Read the model definition and answer for the solid it produces. Units are mm, in the model's axes. A direction names the side the tool comes from. Coordinates: 2 decimals unless noted, no trailing zeros. Write each loop counter-clockwise with the first axis right and the second up, starting at its lowest first coordinate (ties: lowest second). Pieces come first, ordered by that corner, then holes. Notation, with made-up numbers: (41, 26) - (73, 26) arc R30 ccw to (73, 55) - close; hole circle Ø2 at (39, -21). An arc over 180 degrees is marked (long way). Use a Markdown table: item, result.
from build123d import *

# Parameters (mm, degrees)
ESBO_O1_W                  = 170
ESBO_O1_H                  = 30
RESSALTO_EXTRUS_O1_DEPTH   = 150
CORTE_EXTRUS_O1_DEPTH      = 222
CORTE_EXTRUS_O1_DEPTH_BACK = 36
RESSALTO_EXTRUS_O2_DEPTH   = 5
RESSALTO_EXTRUS_O3_DEPTH   = 5
ESBO_O4_W                  = 159.333333333
ESBO_O4_H                  = 140.588235294
CORTE_EXTRUS_O2_DEPTH      = 25
CORTE_EXTRUS_O3_DEPTH      = 31
CORTE_EXTRUS_O4_DEPTH      = 42
FILETE1_R                  = 10
CORTE_EXTRUS_O5_DEPTH      = 32
CORTE_EXTRUS_O6_START      = -15.72292277
CORTE_EXTRUS_O6_OUTLINE_R  = 3.95
CORTE_EXTRUS_O6_DEPTH      = 4.876648775
CORTE_EXTRUS_O7_START      = -132.751356438
CORTE_EXTRUS_O7_OUTLINE_R  = 3.95
CORTE_EXTRUS_O7_DEPTH      = 3.479370229
RESSALTO_EXTRUS_O6_DEPTH   = 17
RESSALTO_EXTRUS_O7_DEPTH   = 4
CORTE_EXTRUS_O8_DEPTH      = 21
F_3DSKETCH12_R             = 1.5
CORTE_EXTRUS_O9_DEPTH      = 14
CORTE_EXTRUS_O10_DEPTH     = 19
ESBO_O11_W                 = 17.407525744
ESBO_O11_H                 = 16.792397695
CORTE_EXTRUS_O11_DEPTH     = 10
CORTE_EXTRUS_O12_DEPTH     = 20
CORTE_EXTRUS_O13_DEPTH     = 14


# Read off the part's stored shape, not the designer's step: Corte-extrusão6, Corte-extrusão7
with BuildPart() as part:
    # Esboço1 → Ressalto-extrusão1 (new body)
    with BuildSketch(Plane(origin=(0, 0, 0), x_dir=(1, 0, 0), z_dir=(0, 1, 0))):
        with Locations((85, 15)):
            Rectangle(ESBO_O1_W, ESBO_O1_H)
        Polygon((80, 160), (0, 30), (170, 30), (170, 160), align=None)
        Polygon((170, 160), (170, 185), (80, 160), align=None)
    extrude(amount=RESSALTO_EXTRUS_O1_DEPTH)

    # Esboço2 → Corte-extrusão1 (cut, two sides: drawn at the far end of the back side and taken through both)
    with BuildSketch(Plane(origin=(0, 0, 0), x_dir=(1, 0, 0), z_dir=(0, 1, 0)).offset(-CORTE_EXTRUS_O1_DEPTH_BACK)):
        Polygon((84.391050739, 157.608625205), (165, 180), (165, 5), (5, 5), (5, 29.866892941), align=None)
    extrude(amount=CORTE_EXTRUS_O1_DEPTH + CORTE_EXTRUS_O1_DEPTH_BACK, mode=Mode.SUBTRACT)

    # Esboço3 → Ressalto-extrusão2 (add)
    with BuildSketch(Plane(origin=(0, 0, 0), x_dir=(1, 0, 0), z_dir=(0, 1, 0))):
        Polygon((84.391050739, 157.608625205), (165, 180), (165, 5), (5, 5), (5, 29.866892941), align=None)
    extrude(amount=RESSALTO_EXTRUS_O2_DEPTH)

    # 3DSketch2 → Ressalto-extrusão3 (add)
    with BuildSketch(Plane(origin=(165, 150, -5), x_dir=(0, 0, -1), z_dir=(0, 1, 0))):
        Polygon((0, 0), (0, 160), (24.866892941, 160), (152.608625205, 80.608949261), (175, 0), align=None)
    extrude(amount=-RESSALTO_EXTRUS_O3_DEPTH)

    # Esboço4 → Corte-extrusão2 (cut)
    with BuildSketch(Plane.XY):
        with Locations((85.333333333, 74.705882353)):
            Rectangle(ESBO_O4_W, ESBO_O4_H)
    extrude(amount=-CORTE_EXTRUS_O2_DEPTH, mode=Mode.SUBTRACT)

    # 3DSketch3 → Corte-extrusão3 (cut)
    with BuildSketch(Plane(origin=(74.759025743, 90, -151.483416833), x_dir=(-0.29071694485714406, -0.8320502943378435, 0.4724150353928592), z_dir=(-0.8516583167045438, 0, -0.5240974256643346))):
        Polygon((0, 0), (22.188007849, 33.282011774), (72.111025509, 0), (49.92301766, -33.282011774), align=None)
    extrude(amount=-CORTE_EXTRUS_O3_DEPTH, mode=Mode.SUBTRACT)

    # 3DSketch4 → Corte-extrusão4 (cut)
    with BuildSketch(Plane(origin=(69.518051487, 130, -142.966833666), x_dir=(-0.37059284368967266, -0.7071067811865471, 0.6022133709956982), z_dir=(0.8516583167045362, 0, 0.5240974256643472))):
        Polygon((0, 0), (14.142135624, -14.142135624), (28.284271247, 0), (14.142135624, 14.142135624), align=None)
    extrude(amount=CORTE_EXTRUS_O4_DEPTH, mode=Mode.SUBTRACT)

    # Filete1
    filete1_edges = [part.edges().sort_by_distance(p)[0] for p in [
        (170, 75, -185),
        (125, 0, -172.5),
        (125, 150, -172.5),
        (80, 75, -160),
        (40, 0, -95),
        (40, 150, -95),
        (0, 75, -30),
        (84.391050739, 75, -157.608625205),
    ]]
    fillet(filete1_edges, radius=FILETE1_R)

    # 3DSketch5 → Corte-extrusão5 (cut)
    with BuildSketch(Plane(origin=(38.121221288, 25, -91.946984593), x_dir=(-0.194644897392922, 0.9284766908852593, 0.31629795826349816), z_dir=(0.851658316704544, 0, 0.5240974256643347))):
        Polygon((0, 0), (14.855627054, 37.139067635), (107.703296143, 0), (92.847669089, -37.139067635), align=None)
    extrude(amount=CORTE_EXTRUS_O5_DEPTH, mode=Mode.SUBTRACT)

    # Corte-extrusão6 outline → Corte-extrusão6 (cut)
    with BuildSketch(Plane(origin=(0, 0, 0), x_dir=(0.5240974256643349, 0, -0.8516583167045437), z_dir=(0.8516583167045437, 0, 0.5240974256643349)).offset(CORTE_EXTRUS_O6_START)):
        with Locations((148.193124726, 20)):
            Circle(CORTE_EXTRUS_O6_OUTLINE_R)
    extrude(amount=CORTE_EXTRUS_O6_DEPTH, mode=Mode.SUBTRACT)

    # Corte-extrusão7 outline → Corte-extrusão7 (cut)
    with BuildSketch(Plane(origin=(0, 0, 0), x_dir=(0.9635179096299408, 0, -0.267643863786094), z_dir=(0.267643863786094, 0, 0.9635179096299409)).offset(CORTE_EXTRUS_O7_START)):
        with Locations((161.993020775, 122.164347625)):
            Circle(CORTE_EXTRUS_O7_OUTLINE_R)
    extrude(amount=CORTE_EXTRUS_O7_DEPTH, mode=Mode.SUBTRACT)

    # 3DSketch9 → Ressalto-extrusão6 (add)
    with BuildSketch(Plane(origin=(76.350750718, 26, -154.069969916), x_dir=(-0.29815073011621673, 0.8224176546598938, 0.4844949364388514), z_dir=(0.8516583167045438, 0, 0.5240974256643349))):
        Polygon((0, 0), (26.758649409, 38.684123705), (82.683049926, 0), (55.924400517, -38.684123705), align=None)
        Polygon((5.017416454, 0.222210211), (27.772783339, 33.118916398), (77.117842619, -1.01413393), (54.362475733, -33.910840117), align=None, mode=Mode.SUBTRACT)
    extrude(amount=RESSALTO_EXTRUS_O6_DEPTH)

    # 3DSketch10 → Ressalto-extrusão7 (add, along a direction that is not the sketch's normal)
    with BuildSketch(Plane(origin=(0, 0, 0), x_dir=(0.7498378553650926, 0.6616216370868463, 0), z_dir=(0, 0, 1))):
        with BuildLine():
            Line((0, 0), (14.996757107, -13.232432742))
            Line((14.996757107, -13.232432742), (28.229189849, 1.764324366))
            ThreePointArc((28.229189849, 1.764324366), (21.556867541, 14.536675999), (25.141622209, 28.493838504))
            Line((25.141622209, 28.493838504), (13.232432742, 14.996757107))
            Line((13.232432742, 14.996757107), (0, 0))
        make_face()
        with BuildLine():
            Line((99.243245563, 112.475678305), (115.742930564, 97.917132715))
            Line((115.742930564, 97.917132715), (100.070543679, 80.155094246))
            ThreePointArc((100.070543679, 80.155094246), (86.055529464, 85.755516688), (71.66166921, 81.216558438))
            Line((71.66166921, 81.216558438), (83.570858678, 94.713639835))
            Line((83.570858678, 94.713639835), (99.243245563, 112.475678305))
        make_face()
        Polygon((226.715680975, 0), (211.718923868, 13.232432742), (198.486491126, -1.764324366), (213.483248233, -14.996757107), align=None)
        Polygon((127.472435412, -112.475678305), (112.475678305, -99.243245563), (125.708111047, -84.246488456), (140.704868154, -97.478921197), align=None)
    extrude(amount=-RESSALTO_EXTRUS_O7_DEPTH, dir=(0.26764386378609445, 0, 0.9635179096299407))

    # 3DSketch11 → Corte-extrusão8 (cut)
    with BuildSketch(Plane(origin=(153.100052242, 17.26943239, -180.305570067), x_dir=(-0.07376023038027929, 0.9970655099962036, 0.02048895288341091), z_dir=(0.2676438637860946, 0, 0.9635179096299407))):
        Polygon((0, 0), (0.269964353, 3.516152018), (46.066103253, 0), (45.7961389, -3.516152018), align=None)
    extrude(amount=CORTE_EXTRUS_O8_DEPTH, mode=Mode.SUBTRACT)

    # 3DSketch12 → Corte-extrusão9 (cut)
    with BuildSketch(Plane(origin=(160, 140, 0), x_dir=(-0.7560654573770964, -0.6544960077503622, 0), z_dir=(0, 0, 1))):
        with Locations(Location((0, 0, 0), (0, 0, 319.118554366))):
            Circle(F_3DSKETCH12_R)
        with Locations(Location((85.084481008, 98.288509459, 0), (0, 0, 319.118554366))):
            Circle(F_3DSKETCH12_R)
        with Locations(Location((113.858951537, -96.124361942, 0), (0, 0, 139.118554366))):
            Circle(F_3DSKETCH12_R)
        with Locations(Location((196.909602971, 0, 0), (0, 0, 139.118554366))):
            Circle(F_3DSKETCH12_R)
    extrude(amount=-CORTE_EXTRUS_O9_DEPTH, mode=Mode.SUBTRACT)

    # 3DSketch13 → Corte-extrusão10 (cut)
    with BuildSketch(Plane(origin=(170, 70.245878967, 0), x_dir=(0, -0.4354246522459521, -0.9002251786172678), z_dir=(-1, 0, 0))):
        Polygon((0, 0), (32.261446294, -15.604350297), (39.809023237, 0), (7.547576943, 15.604350297), align=None)
    extrude(amount=CORTE_EXTRUS_O10_DEPTH, mode=Mode.SUBTRACT)

    # Esboço11 → Corte-extrusão11 (cut)
    with BuildSketch(Plane(origin=(170, 0, 0), x_dir=(0, 0, -1), z_dir=(1, 0, 0))):
        with Locations((8.703762872, 30.096304842)):
            Rectangle(ESBO_O11_W, ESBO_O11_H)
    extrude(amount=-CORTE_EXTRUS_O11_DEPTH, mode=Mode.SUBTRACT)

    # 3DSketch14 → Corte-extrusão12 (cut)
    with BuildSketch(Plane(origin=(170, 87.396079578, 0), x_dir=(0, -0.09341146144778735, -0.9956275904524686), z_dir=(1, 0, 0))):
        Polygon((0, 0), (20.627912038, 1.935345533), (19.506160301, 13.891554783), (-1.121751737, 11.956209249), align=None)
        Polygon((-2.576084268, 27.457236328), (18.165947056, 29.403288726), (16.691971594, 45.113680317), (-4.050059731, 43.167627919), align=None)
        Polygon((91.534016736, 10.656116635), (99.096194716, 11.679615344), (100.676965661, 0), (93.114787682, -1.02349871), align=None)
    extrude(amount=-CORTE_EXTRUS_O12_DEPTH, mode=Mode.SUBTRACT)

    # 3DSketch15 → Corte-extrusão13 (cut)
    with BuildSketch(Plane(origin=(129.748977416, 150, 0), x_dir=(-0.6170578351280018, 0, -0.7869178026370631), z_dir=(0, -1, 0))):
        Polygon((0, 0), (11.819817446, 9.268453377), (19.087630878, 0), (7.267813432, -9.268453377), align=None)
    extrude(amount=CORTE_EXTRUS_O13_DEPTH, mode=Mode.SUBTRACT)


solid = part.part
(1) Each of these flat-tipped pins is pushed along its axis until it touches: P1, Ø3, axis at x = 74, y = 51, coming from the +Z side; P2, Ø12, axis at x = 20, y = 100, coming from the +Z side; P3, Ø1.5, axis at x = 167.5, y = 121.5, coming from the +Z side; P4, Ø12.5, axis at y = 68.5, z = -10.5, coming from the +X side. Where does it stop, or does it pass through?
Report:
| item | result |
|---|---|
| P1 | stops at z = -151.03 |
| P2 | stops at z = -44.35 |
| P3 | stops at z = -20.83 |
| P4 | stops at x = 170 |
(2) For faces 4 (the flat face through (167.535, 83.962, -99.992)), 5 (the flat face through (168, 99.405, -11)), 6 (the flat face through (117.971, 148, -8)), determine the directions among +Z, -Z, +X, -X, +Y, -Y from which every point of the face is accessible in a straight line to the end or side of a thin tool.
Report:
| item | result |
|---|---|
| face 4 | +X |
| face 5 | +Z, +X |
| face 6 | +Z, +Y |
(3) A cutting plane is placed at B-B, the plane y = 50.5. Count the separate pieces of the cut face and the enclosed holes in it, and give its area (3 significant figures).
Report:
| item | result |
|---|---|
| separate pieces | 4 |
| enclosed holes | 0 |
| area | 1,740 mm² |
(4) A cutting plane is placed at A-A, the plane y = 73. Write down the section's boundary in (x, z), and give its area (3 significant figures).
Report:
| item | result |
|---|---|
| outline | (0, -27.17) arc R10 ccw to (1.48, -32.41) - (17.16, -57.88) - (20.96, -55.54) - (5, -29.87) - (5, -5) - (5.67, -5) - (5.67, 0) - (0, 0) - close; (38.12, -91.95) - (53.8, -117.42) - (68.27, -108.51) - (66.18, -105.1) - (55.75, -111.52) - (42.07, -89.52) - close; (74.76, -151.48) - (77.94, -156.66) arc R10 ccw to (83.78, -161.05) - (157.32, -181.48) arc R10 ccw to (170, -171.84) - (170, 0) - (165, 0) - (165, -180) - (88.15, -158.65) arc R10 cw to (82.33, -154.3) - (80.58, -151.47) - (90.83, -145.16) - (89.24, -142.57) - close |
| area | 1,750 mm² |
(5) Straight lines are drawn through the part: L1, parallel to Y at x = 160, z = -1; L2, parallel to X at y = 135, z = -25; L3, parallel to Y at x = 98.5, z = -150. For each, find the intervals that lie inside material, in ascending order.
Report:
| item | result |
|---|---|
| L1 | y = 0 to 8.5, 11.5 to 20, 130.75 to 138.5, 141.5 to 150 |
| L2 | x = 0 to 5, 165 to 170 |
| L3 | y = 0 to 5, 145 to 150 |
(6) The mould has two halves that part along Y. Classify faces 1 (the flat face through (159, 142, 0)), 2 (the cylindrical face through (36.536, 3.007, -83.931)), 3 (the flat face through (30, 25, -74)): pulls with the +Y half, pulls with the -Y half, needs draft (parallel to the pull), parting line crosses it, or undercut.
Report:
| item | result |
|---|---|
| face 1 | needs draft |
| face 2 | pulls with the -Y half |
| face 3 | undercut |
